Input: part model. Units: mm. Frame: model coordinates. A direction names the side the tool comes from. Round coordinates to 2 decimals unless told otherwise and drop trailing zeros. Loops run counter-clockwise (first coordinate to the right, second up) from the corner with the lowest first, then second, coordinate; pieces in that order, holes last. Notation, with made-up numbers: (87, 7) -> (118, 7) arc R13 ccw to (118, 22) -> close; hole circle Ø1 at (21.25, 41.5). An arc over 180 degrees is marked (long way). One line per question, with ' | ' between items. Start each with the question number.
Q1. Contact query for flat-ended pins moving along their axis: P1, Ø7, axis at x = 0, y = 0, coming from the -Z side; P2, Ø8, axis at x = 2.5, y = 4.5, coming from the +Z side; P3, Ø2, axis at x = -3, z = -1.5, coming from the -Y side; P4, Ø1.5, axis at x = 6.5, z = 1.5, coming from the -Y side. Output: stop coordinate, or through.
Q2. Material intervals for L1, parallel to Y at x = 0, z = -1.2; L2, parallel to Y at x = 5.5, z = -0.8; L3, parallel to Z at x = 7, y = 0.25, sorted ascending.
Q3. Access query for faces 4 (the face through (0, 0, 2)), 5 (the face through (0, 0, -1)). Directions: +Z, -Z, +X, -X, +Y, -Y. A direction counts if a zero-diameter tool reaches every point of the face in a straight line with its end or side. Return the directions, or none.
Q4. Cut plane B-B on z = -0.45. Return loops of the section in (x, y).
Q5. Cut plane A-A on z = 0.75. Return loops of the section in (x, y), and give its area (3 significant figures).
Q6. Mould query, pull axis Y, two halves, no side actions, for faces 1 (the face through (-1.73, -7.81, -0.99)), 2 (the face through (-0.59, 4.46, -1.49)), 3 (the face through (3.4, -3.4, -2)). Classes: pulls with the +Y half, pulls with the -Y half, needs draft (parallel to the pull), parting line crosses it, or undercut.
from build123d import *

# Parameters (mm, degrees)
F0_R     = 8
F0_R_2   = 4.5
F2_DEPTH = 2
F3_DEPTH = 1


with BuildPart() as f2:
    # F0 (on Top) → F2 (new body)
    with BuildSketch(Plane.XY):
        Circle(F0_R)
        Circle(F0_R_2, mode=Mode.SUBTRACT)
    extrude(amount=-F2_DEPTH)

    # F0 (on Top) → F3 (join)
    with BuildSketch(Plane.XY):
        Circle(F0_R_2)
    extrude(amount=-F3_DEPTH)

    # F1 (on Front) → F4 (revolve)
    with BuildSketch(Plane.XZ):
        Polygon((0, 2), (0, 0), (8, 0), align=None)
    revolve(axis=Axis((0, 0, 1), (0, 0, 1)))


solid = f2.part
Results:
1) P1: z = -1 | P2: z = 1.71 | P3: y = -7.75 | P4: through
2) L1: -8 to -4.5, 4.5 to 8 | L2: -5.81 to 5.81 | L3: -2 to 0.25
3) face 4: +Z | face 5: -Z
4) outline: circle Ø16 at (0, 0)
5) outline: circle Ø10 at (0, 0) | area: 78.5 mm^2
6) face 1: parting line crosses it | face 2: undercut | face 3: needs draft
